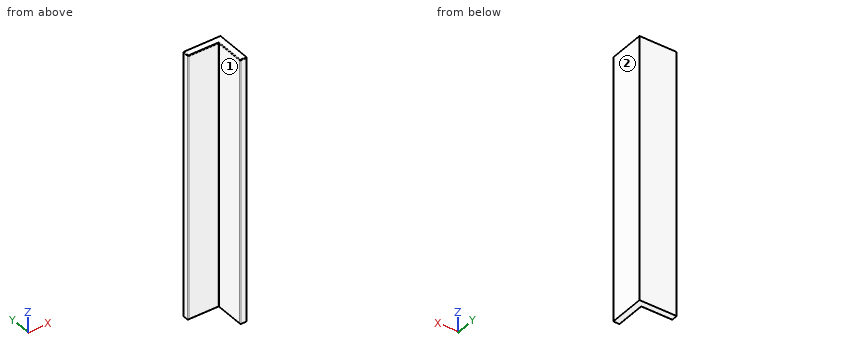
```python
from build123d import *

# Parameters (mm, degrees)
F0_W      = 38.9711558819
F0_H      = 53.4048825502
F1_DEPTH  = 18
F2_DEPTH  = 50
F3_DEPTH  = 25
F4_DEPTH  = 718
F5_W      = 25
F5_H      = 718
F6_DEPTH  = 20
F7_DEPTH  = 7
F8_DEPTH  = 80
F9_DEPTH  = 20
F10_DEPTH = 70
F11_DEPTH = 18
F12_DEPTH = 1
F13_R     = 2


with BuildPart() as f1:
    # F0 (on Front) → F1 (new body)
    with BuildSketch(Plane.XZ):
        with Locations((19.4855779409, 26.7024412751)):
            Rectangle(F0_W, F0_H)
    extrude(amount=F1_DEPTH)

    # F2 (add): a face of the model
    f2_faces = [f1.faces().sort_by_distance(p)[0] for p in [
        (0, -9, 26.7024412751),
    ]]
    extrude(f2_faces, amount=-F2_DEPTH)

    # F3 (add): a face of the model
    f3_faces = [f1.faces().sort_by_distance(p)[0] for p in [
        (25, -9, 0),
    ]]
    extrude(f3_faces, amount=-F3_DEPTH)

    # F4 (add): a face of the model
    f4_faces = [f1.faces().sort_by_distance(p)[0] for p in [
        (25, -9, 0),
    ]]
    extrude(f4_faces, amount=-F4_DEPTH)

    # F5 (on face) → F6 (join)
    with BuildSketch(Plane.XZ.offset(18)):
        with Locations((37.5, 359)):
            Rectangle(F5_W, F5_H)
    extrude(amount=F6_DEPTH)

    # F7 (cut): a face of the model
    f7_faces = [f1.faces().sort_by_distance(p)[0] for p in [
        (25, -28, 359),
    ]]
    extrude(f7_faces, amount=-F7_DEPTH, mode=Mode.SUBTRACT)

    # F8 (add): a face of the model
    f8_faces = [f1.faces().sort_by_distance(p)[0] for p in [
        (41, -38, 359),
    ]]
    extrude(f8_faces, amount=F8_DEPTH)

    # F9 (cut): a face of the model
    f9_faces = [f1.faces().sort_by_distance(p)[0] for p in [
        (41, -118, 359),
    ]]
    extrude(f9_faces, amount=-F9_DEPTH, mode=Mode.SUBTRACT)

    # F10 (add): a face of the model
    f10_faces = [f1.faces().sort_by_distance(p)[0] for p in [
        (0, -9, 359),
    ]]
    extrude(f10_faces, amount=F10_DEPTH)

    # F11 (cut): a face of the model
    f11_faces = [f1.faces().sort_by_distance(p)[0] for p in [
        (-70, -9, 359),
    ]]
    extrude(f11_faces, amount=-F11_DEPTH, mode=Mode.SUBTRACT)

    # F12 (cut): a face of the model
    f12_faces = [f1.faces().sort_by_distance(p)[0] for p in [
        (-52, -9, 359),
    ]]
    extrude(f12_faces, amount=-F12_DEPTH, mode=Mode.SUBTRACT)

    # F13
    f13_edges = [f1.edges().sort_by_distance(p)[0] for p in [
        (-9.5, -18, 0),
        (-51, -18, 359),
        (-9.5, -18, 718),
        (32, -18, 359),
        (32, -58, 0),
        (32, -98, 359),
        (32, -58, 718),
        (41, -98, 718),
        (-51, -9, 718),
    ]]
    fillet(f13_edges, radius=F13_R)


solid = f1.part
```
Geometry: final body of the model. Coordinates: model frame, mm. Face numbers are marked on the shaded views. A direction names the side the tool comes from. Round coordinates to 2 decimals unless told otherwise and drop trailing zeros. Order: outer loops, then holes, each group sorted by start corner. A loop starts at its lowest first (then second) coordinate and runs counter-clockwise, first axis right, second up. Notation, with made-up numbers: (76.5, 43) - (108.5, 43) arc R20 cw to (108.5, 53) - close; hole circle Ø1 at (-20.75, 27). An arc over 180 degrees is marked (long way). Use CSV: the item, a comma, the result in double quotes. Start each with the question number.
Q1. Section query A-A (z = 645). Return loops of the section in (x, y).
Q2. Section query C-C (y = -42). Return loops of the section in (x, z), and give its area (3 significant figures).
Q3. First-contact query: pin 1 (3 mm diameter, centred on x = -16, z = 109, fed in from -Y); pin 2 (4 mm diameter, centred on y = -29.5, z = 295.5, fed in from -X); pin 3 (4 mm diameter, centred on x = 28.5, y = -66, fed in from +Z). Flat tips, straight axial feed; report the tip coordinate or a pass-through.
Q4. Section query B-B (x = 14). Return loops of the section in (y, z), and give its area (3 significant figures).
Q5. Access query for the marked faces 1 and 2. Directions: +Z, -Z, +X, -X, +Y, -Y. A direction counts if a zero-diameter tool reaches every point of the face in a straight line with its end or side. Return the directions, or none.
Q6. Material intervals for line 1 along Y through (x, z) = (-15.5, 589.5); line 2 along X through (y, z) = (-60, 577); line 3 along Y through (x, z) = (31, 75.5), sorted ascending. Write a range as from..to.
Result set:
1,outline,"(-51, -16) arc R2 ccw to (-49, -18) - (30, -18) arc R2 cw to (32, -20) - (32, -96) arc R2 ccw to (34, -98) - (50, -98) - (50, 0) - (-51, 0) - close"
2,outline,"(32, 2) arc R2 ccw to (34, 0) - (50, 0) - (50, 718) - (34, 718) arc R2 ccw to (32, 716) - close"
2,area,"12,900 mm2"
3,pin 1,"stops at y = -18"
3,pin 2,"stops at x = 32"
3,pin 3,"passes through"
4,outline,"(-18, 2) arc R2 ccw to (-16, 0) - (0, 0) - (0, 718) - (-16, 718) arc R2 ccw to (-18, 716) - close"
4,area,"12,900 mm2"
5,face 1,"+Z, -Z, -X, -Y"
5,face 2,"+Z, -Z, +X, +Y, -Y"
6,line 1,"y = -18..0"
6,line 2,"x = 32..50"
6,line 3,"y = -18.27..0"
